Input: part model. Units: mm. Frame: model coordinates. Face numbers are marked on the shaded views. A direction names the side the tool comes from. Give positions to 0.01 mm unless a question says otherwise; leave off trailing zeros. Loops run counter-clockwise (first coordinate to the right, second up) from the corner with the lowest first, then second, coordinate; pieces in that order, holes last. Notation, with made-up numbers: M -17.75,45 L -11.75,45 A11 ccw -11.75,63 Z; hole C 7,-17.75 d9. An arc over 180 degrees is marked long. One line per item, written item: value. Start each with the question number.
(1) Ray query, line 1 along Z through (x, y) = (-5.75, 0); line 2 along Y through (x, z) = (-3.5, 4). Return the intervals inside material, ascending. Write a range as from..to.
(2) Access query for the marked faces 5, 6 and 7. Directions: +Z, -Z, +X, -X, +Y, -Y. A direction counts if a zero-diameter tool reaches every point of the face in a straight line with its end or side. Return the directions, or none.
(3) Section C-C on x = -37. Output: boundary loops of the cut face in (y, z).
(4) Section A-A on z = 0. Output: boundary loops of the cut face in (x, y).
(5) Section D-D on z = -24. Output: boundary loops of the cut face in (x, y), plus the area to 3 significant figures.
(6) Pull-direction query (Z, two-part tool) for the marked faces 1, 2, 3 and 4; classes: released by +Z, released by -Z, zero draft, split by the parting line, or undercut.
(7) Pin query (flat end, axial travel): P1, Ø1.5, axis at x = -8, z = 36, coming from the -Y side; P2, Ø11, axis at y = 0, z = 0, coming from the +X side; P3, Ø12, axis at x = -11, y = -16, coming from the -Z side; P4, Ø5, axis at x = -15.5, y = 28, coming from the +Z side. Return the tip coordinate at first contact, or that it passes through.
Autodesk Inventor part; units mm, degrees
ref_plane "YZ Plane" through (0, 0, 0) normal (1, 0, 0) x (0, 1, 0)
ref_plane "XZ Plane" through (0, 0, 0) normal (0, 1, 0) x (-1, 0, 0)
ref_plane "XY Plane" through (0, 0, 0) normal (0, 0, 1) x (1, 0, 0)
sketch "Sketch1" plane through (0, 0, 0) normal (0, 1, 0) x (-1, 0, 0)
  line L0 (0, 0) -> (0, -6) construction
  line L1 (0, -6) -> (40, -6)
  line L2 (40, -6) -> (40, -50) construction
  line L3 (40, -50) -> (0, -50)
  line L4 (0, -50) -> (0, -35)
  line L5 (0, -35) -> (10, -35)
  line L6 (10, -35) -> (10, -15)
  line L7 (10, -15) -> (0, -15)
  line L8 (0, -15) -> (0, -6)
  line L9 (20, -6) -> (20, -50) construction
  line L10 (40, -50) -> (40, -35)
  line L11 (40, -35) -> (30, -35)
  line L12 (30, -35) -> (30, -15)
  line L13 (30, -15) -> (40, -15)
  line L14 (40, -15) -> (40, -6)
  line L15 (0, 0) -> (40, 0) construction
  dimension "d0" = 6
  dimension "d1" = 40
  dimension "d2" = 44
  dimension "d3" = 15
  dimension "d4" = 10
  dimension "d5" = 20
revolve "Revolution1" add sketch "Sketch1" angle 360 about axis through (0, 0, 0) along (-1, 0, 0)
properties part number "KZ"
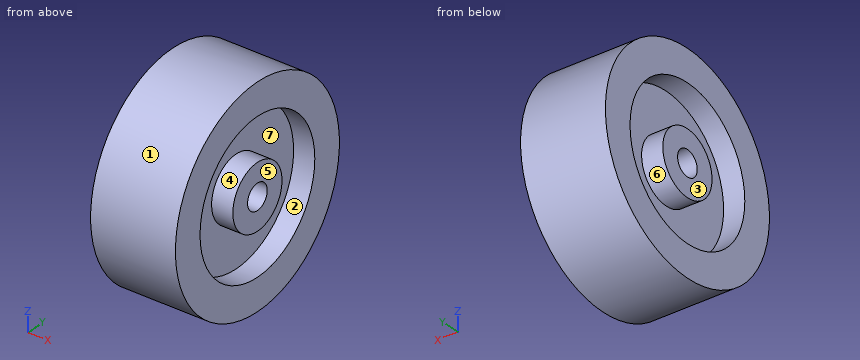
Output values:
1. line 1: z = -50..-35, -15..-6, 6..15, 35..50
1. line 2: y = -49.84..-34.77, -14.46..-4.47, 4.47..14.46, 34.77..49.84
2. face 5: +Z, -Z, +X, +Y, -Y
2. face 6: -X
2. face 7: +X
3. outline: C 0,0 d100; C 0,0 d30; hole C 0,0 d70; hole C 0,0 d12
4. outline: M -40,-50 L 0,-50 L 0,-35 L -10,-35 L -10,-15 L 0,-15 L 0,-6 L -40,-6 L -40,-15 L -30,-15 L -30,-35 L -40,-35 Z; M -40,6 L 0,6 L 0,15 L -10,15 L -10,35 L 0,35 L 0,50 L -40,50 L -40,35 L -30,35 L -30,15 L -40,15 Z
5. outline: M -40,-43.86 L 0,-43.86 L 0,-25.48 L -10,-25.48 L -10,25.48 L 0,25.48 L 0,43.86 L -40,43.86 L -40,25.48 L -30,25.48 L -30,-25.48 L -40,-25.48 Z
5. area: 2,490 mm²
6. face 1: split by the parting line
6. face 2: undercut
6. face 3: zero draft
6. face 4: undercut
7. P1: stops at y = -35.46
7. P2: passes through
7. P3: stops at z = -48.99
7. P4: stops at z = 43.01
